```python
from build123d import *

# Parameters (mm, degrees)
BOSS_EXTRUDE1_DEPTH       = 50.8
F_97_0_5_DIAMETER_HOLE1_D = 12.7
F_97_0_5_DIAMETER_HOLE2_D = 12.7


with BuildPart() as part:
    # Sketch1 → Boss-Extrude1 (new body)
    with BuildSketch(Plane.XY):
        Polygon((0, 0), (0, 38.1), (2.54, 38.1), (2.54, 2.54), (38.1, 2.54), (38.1, 0), align=None)
    extrude(amount=BOSS_EXTRUDE1_DEPTH)

    # #97 (0.5) Diameter Hole1 (through all)
    with Locations(Plane(origin=(2.54, 19.05, 25.4), x_dir=(0, 1, 0), z_dir=(1, 0, 0))):
        with Locations((0, 0)):
            Hole(F_97_0_5_DIAMETER_HOLE1_D / 2)

    # #97 (0.5) Diameter Hole2 (through all)
    with Locations(Plane(origin=(0, 2.54, 0), x_dir=(1, 0, 0), z_dir=(0, 1, 0))):
        with Locations((19.05, -25.4)):
            Hole(F_97_0_5_DIAMETER_HOLE2_D / 2)


solid = part.part
```
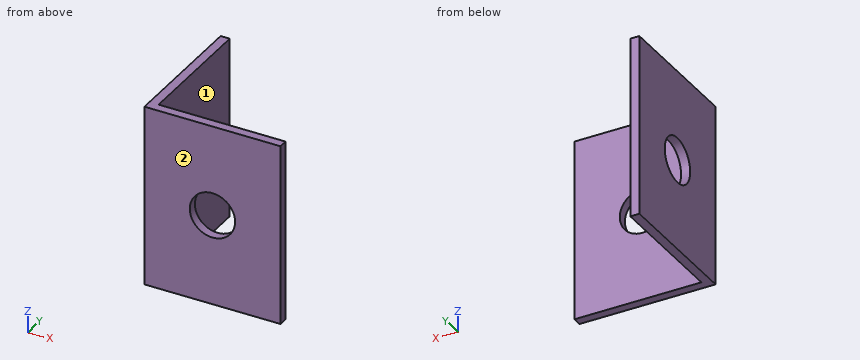
Model file for the job. Use its own axes, mm. Face numbers are marked on the shaded views. A direction names the side the tool comes from. Give positions to 0.01 mm unless a question says otherwise; leave off trailing zeros. Write each loop counter-clockwise with the first axis right and the second up, starting at its lowest first coordinate (ties: lowest second). Pieces come first, ordered by that corner, then holes. Notation, with made-up numbers: M 70.25,42.5 L 80.25,42.5 A11 cw 80.25,63.5 Z; hole C 2,-7 d10. An arc over 180 degrees is marked long. Use a Markdown table: item, result.
1) Cut at B-B (z = 25.4). List the corners of the cut face in (x, y).
Responses:
| item | result |
|---|---|
| outline | M 0,0 L 12.7,0 L 12.7,2.54 L 2.54,2.54 L 2.54,12.7 L 0,12.7 Z; M 0,25.4 L 2.54,25.4 L 2.54,38.1 L 0,38.1 Z; M 25.4,0 L 38.1,0 L 38.1,2.54 L 25.4,2.54 Z |
2) Pin check, flat tips, straight feed: pin 1 (10 mm diameter, centred on x = 19.05, z = 25.4, fed in from +Y); pin 2 (12 mm diameter, centred on y = 19.5, z = 30.5, fed in from +X); pin 3 (8 mm diameter, centred on x = 29.5, z = 41.5, fed in from +Y). Stop position of each tip, or through.
Responses:
| item | result |
|---|---|
| pin 1 | passes through |
| pin 2 | stops at x = 2.54 |
| pin 3 | stops at y = 2.54 |
3) Tool access for the marked faces 1 and 2: list every direction of +Z, -Z, +X, -X, +Y, -Y with a clear straight run to the whole face (end or side of a thin tool).
Responses:
| item | result |
|---|---|
| face 1 | +Z, -Z, +X, +Y |
| face 2 | +Z, -Z, +X, -X, -Y |
4) Cut at D-D (z = 34). List the corners of the cut face in (x, y).
Responses:
| item | result |
|---|---|
| outline | M 0,0 L 38.1,0 L 38.1,2.54 L 2.54,2.54 L 2.54,38.1 L 0,38.1 Z |
5) Cut at A-A (y = 19.05). List the corners of the cut face in (x, z).
Responses:
| item | result |
|---|---|
| outline | M 0,0 L 2.54,0 L 2.54,19.05 L 0,19.05 Z; M 0,31.75 L 2.54,31.75 L 2.54,50.8 L 0,50.8 Z |
6) Drill centre lines: line 1 (Z direction, x = 1, y = 19); line 2 (Y direction, x = 1, z = 25); line 3 (X direction, y = 1.05, z = 25.4). Where is each one in solid material? Low to high. Write a range as from..to.
Responses:
| item | result |
|---|---|
| line 1 | z = 0..19.05, 31.75..50.8 |
| line 2 | y = 0..12.71, 25.39..38.1 |
| line 3 | x = 0..12.7, 25.4..38.1 |
